For this review, take the finished solid that the model builds, in its own axes (mm). A direction names the side the tool comes from. Round coordinates to 2 decimals unless told otherwise and drop trailing zeros. Loops run counter-clockwise (first coordinate to the right, second up) from the corner with the lowest first, then second, coordinate; pieces in that order, holes last. Notation, with made-up numbers: M 4,-21.75 L 8,-21.75 A7 ccw 8,-12.75 Z; hole C 55.25,11 d2. An arc over 180 degrees is marked long. One line per question, with ' | ' between items. Start each with the question number.
1) For probe 1 along X at (y, z) = (45.6, 0); probe 2 along Y at (x, z) = (-2.5, -2.5); probe 3 along Z at (x, y) = (2.75, 18), list the stretches that pass through material, from the lowest coordinate up. Write a range as from..to.
2) We need section D-D (y = 47.5). Give the boundary of the cut face in (x, z).
3) For pin 1 Ø1.5 at (x, y) = (5, 19) entering from -Z; pin 2 Ø2.5 at (x, z) = (-8, 0) entering from +Y; pin 3 Ø4 at (y, z) = (48, 8) entering from -X, all flat-tipped, find the tip position at first contact; note any pin that passes through.
4) We need section B-B (y = 29). Give the boundary of the cut face in (x, z) (3 decimals).
5) For faces 5 (the face through (5, 16.5, -6)), 6 (the face through (11, -2, 0)), 7 (the face through (0, -4, 0)), 8 (the face through (13.687, 6.803, -0.602)), list the 3-axis set-ups (+Z, -Z, +X, -X, +Y, -Y) from which the entire face can be reached by the end or side of a thin tool; tool diameter is ignored.
6) Mouldability with a two-part tool opening along X and no side actions: class faces 1 (the face through (0, 46.5, -6)), 2 (the face through (-11.5, -2, 0)), 3 (the face through (11.5, -2, 0)), 4 (the face through (-3.116, 27.844, 14.033)) as pulls with the +X half, pulls with the -X half, needs draft (parallel to the pull), parting line crosses it, or undercut.
7) We need section C-C (z = -10.65). Give the boundary of the cut face in (x, y).
Autodesk Inventor part; units mm, degrees
ref_plane "Work Plane1" through (0, 41.5, 0) normal (0, 1, 0) x (1, 0, 0)
ref_plane "Work Plane2" through (0, 50.2, 0) normal (0, 1, 0) x (1, 0, 0)
ref_plane "YZ Plane" through (0, 0, 0) normal (1, 0, 0) x (0, 1, 0)
sketch "Sketch1" plane through (0, 0, 0) normal (0, 1, 0) x (-1, 0, 0)
  circle A0 centre (0, 0) radius 13.7
  dimension "d0" = 27.4
extrude "Extrusion1" add sketch "Sketch1" along normal blind 46.5
sketch "Sketch2" plane through (0, 46.5, 0) normal (0, 1, 0) x (1, 0, 0)
  circle A0 centre (0, 0) radius 13.7
  circle A1 centre (0, 0) radius 5
  dimension "d3" = 10
extrude "Extrusion2" add sketch "Sketch2" along normal blind 2.7 contours A1
sketch "Sketch3" plane through (0, 46.5, 0) normal (0, 1, 0) x (1, 0, 0)
  circle A0 centre (0, 0) radius 5
  circle A1 centre (0, 0) radius 5
  circle A2 centre (0, 0) radius 13.7
  circle A3 centre (0, 0) radius 13.7
  line L0 (-13.7, 0) -> (13.7, 0)
  point P0 (-8, 0)
  point P1 (8, 0)
  dimension "d6" = 16
  dimension "d7" = 5.7
  dimension "d8" = 5.7
hole "Hole1" at (-8, 46.5, 0) at (8, 46.5, 0) direction (0, -1, 0) diameter 2.1129 depth 2.8
ref_plane "Work Plane1" through (0, 41.5, 0) normal (0, 1, 0) x (1, 0, 0)
sketch "Sketch4" plane through (0, 41.5, 0) normal (0, 1, 0) x (1, 0, 0)
  circle A0 centre (0, 0) radius 14.375
  dimension "d17" = 28.75
extrude "Extrusion3" add sketch "Sketch4" against normal blind 27.7
sketch "Sketch5" plane through (0, 0, 0) normal (0, -1, 0) x (1, 0, 0)
  circle A0 centre (0, 0) radius 5
  dimension "d20" = 10
extrude "Extrusion4" add sketch "Sketch5" along normal blind 4
sketch "Sketch6" plane through (0, 0, 0) normal (0, -1, 0) x (1, 0, 0)
  circle A0 centre (0, 0) radius 5
  circle A1 centre (0, 0) radius 5
  circle A2 centre (0, 0) radius 13.7
  circle A3 centre (0, 0) radius 13.7
  line L0 (13.7, 0) -> (-13.7, 0)
  line L1 (-11.5, 1.5) -> (-12, 1.5)
  line L2 (-12, 1.5) -> (-12, -1.5)
  line L3 (-12, -1.5) -> (-11.5, -1.5)
  line L4 (-11.5, -1.5) -> (-11.5, 1.5)
  line L5 (11.5, 1.5) -> (11, 1.5)
  line L6 (11, 1.5) -> (11, -1.5)
  line L7 (11, -1.5) -> (11.5, -1.5)
  line L8 (11.5, -1.5) -> (11.5, 1.5)
  dimension "d23" = 22.5
  dimension "d24" = 0.5
  dimension "d25" = 0.5
  dimension "d26" = 11.5
  dimension "d27" = 11.5
  dimension "d28" = 3
  dimension "d29" = 3
  dimension "d30" = 1.5
  dimension "d31" = 1.5
extrude "Extrusion5" add sketch "Sketch6" along normal up to surface (4 mm away) contours L6 L5 L8 L0 | L0 L8 L7 L6 | L4 L3 L2 L0 | L0 L2 L1 L4
sketch "Sketch7" plane through (0, 49.2, 0) normal (0, 1, 0) x (1, 0, 0)
  circle A0 centre (0, 0) radius 1.1
  dimension "d34" = 2.2
extrude "Extrusion6" add sketch "Sketch7" along normal blind 13.5
ref_plane "Work Plane2" through (0, 50.2, 0) normal (0, 1, 0) x (1, 0, 0)
sketch "Sketch10" plane through (0, 0, 0) normal (1, 0, 0) x (0, 1, 0)
  line L0 (0, -13.7) -> (0, 13.7)
  line L1 (13.8, 13.7) -> (13.8, -13.7)
  line L2 (9, 4.6) -> (13.8, 4.6)
  line L3 (13.8, 4.6) -> (13.8, -4.6)
  line L4 (13.8, -4.6) -> (9, -4.6)
  line L5 (9, -4.6) -> (9, 4.6)
  circle A0 centre (11.4, 4.6) radius 2.4
  circle A1 centre (11.4, -4.6) radius 2.4
  line L6 (0, 0) -> (13.8, 0)
  line L7 (13.8, 13.7) -> (13.8, -13.7)
  line L8 (0, -13.7) -> (13.8, -13.7)
  point P0 (11.4, 7)
  point P1 (11.4, -7)
  point P2 (13.8, -4.6)
  dimension "d57" = 9
  dimension "d59" = 0
  dimension "d60" = 4.8
  dimension "d61" = 13.8
  dimension "d62" = 2.4
  dimension "d63" = 2.4
  dimension "d64" = 14
  dimension "d65" = 4.6
  dimension "d66" = 4.6
  dimension "d69" = 6.7
extrude "Extrusion9" cut sketch "Sketch10" along normal mid plane 31.5 contours L6 L1 A1 L5 | L5 A0 L1 L6 | A1 L4 | L4 A1 | A0 L2 | L2 A0
sketch "Sketch11" plane through (0, 46.5, 0) normal (0, 1, 0) x (1, 0, 0)
  circle A0 centre (-8, 0) radius 1.0564
  circle A1 centre (8, 0) radius 1.0564
  circle A2 centre (0, 0) radius 5
  circle A3 centre (0, 0) radius 13.7
  circle A4 centre (8, 0) radius 1.0564
  circle A5 centre (0, 0) radius 13.7
  line L0 (13.7, 0) -> (-13.7, 0)
  circle A6 centre (0, 0) radius 1.1
  circle A7 centre (0, 0) radius 9.0564
  circle A8 centre (0, 0) radius 6.9436
  circle A9 centre (8, 0) radius 1.0564
  line L1 (1.8876, -9.0564) -> (-1.9124, -9.0564)
  line L2 (-1.9124, -9.0564) -> (-1.9124, 9.0564)
  line L3 (-1.9124, 9.0564) -> (1.8876, 9.0564)
  line L4 (1.8876, 9.0564) -> (1.8876, -9.0564)
  line L5 (-0.0124, -13.7) -> (-0.0124, 13.7)
  line L6 (9.0564, -3.15) -> (-9.0564, -3.15)
  line L7 (-9.0564, -3.15) -> (-9.0564, 3.15)
  line L8 (-9.0564, 3.15) -> (9.0564, 3.15)
  line L9 (9.0564, 3.15) -> (9.0564, -3.15)
  circle A10 centre (6.8048, -4.2064) radius 1.0564
  circle A11 centre (2.9441, -7.4386) radius 1.0564
  circle A12 centre (-2.9688, -7.4287) radius 1.0564
  circle A13 centre (-6.8048, -4.2064) radius 1.0564
  circle A14 centre (-6.8048, 4.2064) radius 1.0564
  line L10 (-11.7767, 7) -> (11.7767, 7)
  circle A15 centre (-2.9688, 7.4287) radius 1.0564
  circle A16 centre (2.9441, 7.4386) radius 1.0564
  circle A17 centre (6.8048, 4.2064) radius 1.0564
  circle A18 centre (-0.0124, 10.65) radius 1.15
  point P0 (9.0564, 0)
  point P1 (7.8048, -3.2064)
  point P2 (3.3328, 8.4209)
  point P3 (2.5553, 6.4563)
  point P4 (5.9062, 3.651)
  point P5 (7.7035, 4.7619)
  point P6 (-5.9062, 3.651)
  point P7 (-2.5768, 6.4477)
  point P8 (-3.3608, 8.4097)
  point P9 (-7.7035, 4.7619)
  point P10 (-3.3608, -8.4097)
  point P11 (-2.5768, -6.4477)
  point P12 (-5.9062, -3.651)
  point P13 (-7.7035, -4.7619)
  point P14 (7.7035, -4.7619)
  point P15 (5.9062, -3.651)
  point P16 (2.5553, -6.4563)
  point P17 (3.3328, -8.4209)
  point P18 (-0.0124, 11.8)
  dimension "d78" = 2.3
  dimension "d70" = 3.8
  dimension "d71" = 1.9
  dimension "d72" = 1.9
  dimension "d73" = 6.3
  dimension "d74" = 3.15
  dimension "d75" = 3.15
  dimension "d79" = 1.9
extrude "Extrusion10" cut sketch "Sketch11" against normal blind 30 contours A14 A7 L10 A15 A8 | A14 | A8 A12 A7 A13 | A13 | A15 L10 | A12 | A7 A15 L10 | A15 L10 | A18 L5 | L5 A18 | L10 A16 A7 | A7 A17 A8 A16 L10 | A11 A8 A10 A7 | A11 | A17 | A16 L10 | A16 L10 | A10
equation "\"d26\" = d27"
equation "\"d30\" = d31"
equation "\"d65\" = d66"
equation "\"d71\" = d72"
equation "\"d74\" = d75"
equation "\"d41\" = d42"
properties part number "rs390" material "Steel, Mild"
Answers below:
1) probe 1: -13.7..-9.06, -6.94..6.94, 9.06..13.7 | probe 2: -4..9, 13.8..49.2 | probe 3: -14.11..-8.48, -6.38..6.38, 8.48..14.11
2) outline: C 0,0 d10
3) pin 1: z = -13.73 | pin 2: y = 46.5 | pin 3: x = -11.96
4) outline: C 0,0 d28.75; hole M -7.703,-4.762 A9.056 ccw -3.361,-8.41 A1.056 ccw -2.577,-6.448 A6.944 cw -5.906,-3.651 A1.056 ccw Z; hole M -7.703,4.762 A1.056 ccw -5.906,3.651 A6.944 cw -2.577,6.448 A1.056 ccw -3.361,8.41 A9.056 ccw Z; hole C -0.012,-10.65 d2.3; hole M 2.555,-6.456 A1.056 ccw 3.333,-8.421 A9.056 ccw 7.703,-4.762 A1.056 ccw 5.906,-3.651 A6.944 cw Z; hole M 2.555,6.456 A6.944 cw 5.906,3.651 A1.056 ccw 7.703,4.762 A9.056 ccw 3.333,8.421 A1.056 ccw Z
5) face 5: +Y | face 6: +Z, -Z, -Y | face 7: +Z, -Z, +X, -X, -Y | face 8: -Y
6) face 1: needs draft | face 2: undercut | face 3: pulls with the +X half | face 4: parting line crosses it
7) outline: M -9.65,13.8 L -8.62,13.8 L -8.62,0 L 8.62,0 L 8.62,13.8 L 9.65,13.8 L 9.65,41.5 L 8.62,41.5 L 8.62,46.5 L 1.14,46.5 L 1.14,16.5 L -1.16,16.5 L -1.16,46.5 L -8.62,46.5 L -8.62,41.5 L -9.65,41.5 Z
